from build123d import *

# Parameters (mm, degrees)
SKETCH1_R           = 44.45
BOSS_EXTRUDE1_DEPTH = 25.4
CHAMFER1_SIZE       = 10
SKETCH3_R           = 1.8161
CUT_EXTRUDE1_DEPTH  = 26.4
BOSS_EXTRUDE3_DEPTH = 50.8


with BuildPart() as part:
    # Sketch1 → Boss-Extrude1 (new body)
    with BuildSketch(Plane.XY):
        with BuildLine():
            ThreePointArc((67.188694676, -58.214167586), (88.9, 0), (67.188694676, 58.214167586))
            ThreePointArc((67.188694676, 58.214167586), (67.351920908, 67.351920908), (58.214167586, 67.188694676))
            ThreePointArc((58.214167586, 67.188694676), (0, 88.9), (-58.214167586, 67.188694676))
            ThreePointArc((-58.214167586, 67.188694676), (-67.351920908, 67.351920908), (-67.188694676, 58.214167586))
            ThreePointArc((-67.188694676, 58.214167586), (-88.9, 0), (-67.188694676, -58.214167586))
            ThreePointArc((-67.188694676, -58.214167586), (-67.351920908, -67.351920908), (-58.214167586, -67.188694676))
            ThreePointArc((-58.214167586, -67.188694676), (0, -88.9), (58.214167586, -67.188694676))
            ThreePointArc((58.214167586, -67.188694676), (67.351920908, -67.351920908), (67.188694676, -58.214167586))
        make_face()
        Circle(SKETCH1_R, mode=Mode.SUBTRACT)
    extrude(amount=BOSS_EXTRUDE1_DEPTH)

    # Chamfer1
    chamfer1_edges = [part.edges().sort_by_distance(p)[0] for p in [
        (-44.45, 0, 25.4),
    ]]
    chamfer(chamfer1_edges, length=CHAMFER1_SIZE)

    # Sketch3 → Cut-Extrude1 (cut, through all)
    with BuildSketch(Plane.XY.offset(25.4)):
        with Locations((61.065741623, 61.065741623)):
            Circle(SKETCH3_R)
        with Locations((61.065741623, -61.065741623)):
            Circle(SKETCH3_R)
        with Locations((-61.065741623, -61.065741623)):
            Circle(SKETCH3_R)
        with Locations((-61.065741623, 61.065741623)):
            Circle(SKETCH3_R)
    extrude(amount=-CUT_EXTRUDE1_DEPTH, mode=Mode.SUBTRACT)

    # Sketch5 → Boss-Extrude3 (add)
    with BuildSketch(Plane(origin=(0, 0, 0), x_dir=(-1, 0, 0), z_dir=(0, 0, -1))):
        with BuildLine():
            Line((-76.835, 12.7), (-56.515, 12.7))
            ThreePointArc((-56.515, 12.7), (-54.718948776, 11.956051224), (-53.975, 10.16))
            Line((-53.975, 10.16), (-53.975, -10.16))
            ThreePointArc((-53.975, -10.16), (-54.718948776, -11.956051224), (-56.515, -12.7))
            Line((-56.515, -12.7), (-76.835, -12.7))
            ThreePointArc((-76.835, -12.7), (-78.631051224, -11.956051224), (-79.375, -10.16))
            Line((-79.375, -10.16), (-79.375, 10.16))
            ThreePointArc((-79.375, 10.16), (-78.631051224, 11.956051224), (-76.835, 12.7))
        make_face()
        with BuildLine():
            Line((-10.16, -79.375), (10.16, -79.375))
            ThreePointArc((10.16, -79.375), (11.956051224, -78.631051224), (12.7, -76.835))
            Line((12.7, -76.835), (12.7, -56.515))
            ThreePointArc((12.7, -56.515), (11.956051224, -54.718948776), (10.16, -53.975))
            Line((10.16, -53.975), (-10.16, -53.975))
            ThreePointArc((-10.16, -53.975), (-11.956051224, -54.718948776), (-12.7, -56.515))
            Line((-12.7, -56.515), (-12.7, -76.835))
            ThreePointArc((-12.7, -76.835), (-11.956051224, -78.631051224), (-10.16, -79.375))
        make_face()
        with BuildLine():
            Line((12.7, 76.835), (12.7, 56.515))
            ThreePointArc((12.7, 56.515), (11.956051224, 54.718948776), (10.16, 53.975))
            Line((10.16, 53.975), (-10.16, 53.975))
            ThreePointArc((-10.16, 53.975), (-11.956051224, 54.718948776), (-12.7, 56.515))
            Line((-12.7, 56.515), (-12.7, 76.835))
            ThreePointArc((-12.7, 76.835), (-11.956051224, 78.631051224), (-10.16, 79.375))
            Line((-10.16, 79.375), (10.16, 79.375))
            ThreePointArc((10.16, 79.375), (11.956051224, 78.631051224), (12.7, 76.835))
        make_face()
        with BuildLine():
            Line((76.835, -12.7), (56.515, -12.7))
            ThreePointArc((56.515, -12.7), (54.718948776, -11.956051224), (53.975, -10.16))
            Line((53.975, -10.16), (53.975, 10.16))
            ThreePointArc((53.975, 10.16), (54.718948776, 11.956051224), (56.515, 12.7))
            Line((56.515, 12.7), (76.835, 12.7))
            ThreePointArc((76.835, 12.7), (78.631051224, 11.956051224), (79.375, 10.16))
            Line((79.375, 10.16), (79.375, -10.16))
            ThreePointArc((79.375, -10.16), (78.631051224, -11.956051224), (76.835, -12.7))
        make_face()
    extrude(amount=BOSS_EXTRUDE3_DEPTH)


solid = part.part
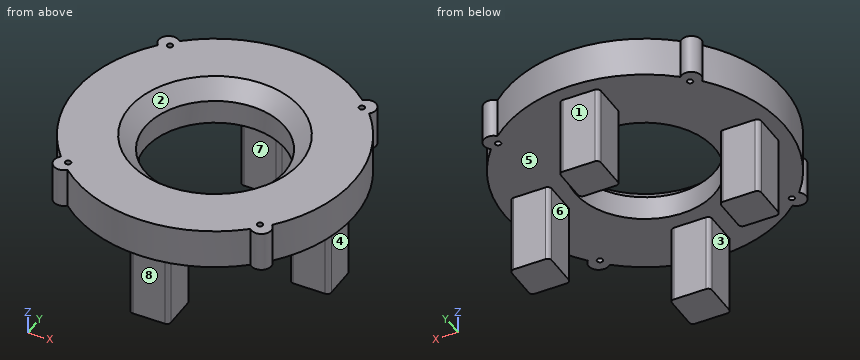
The model under review builds one solid part; all positions refer to its coordinate system, in mm. Face numbers are marked on the shaded views. A direction names the side the tool comes from. Give positions to 0.01 mm unless a question says otherwise; leave off trailing zeros. Loops run counter-clockwise (first coordinate to the right, second up) from the corner with the lowest first, then second, coordinate; pieces in that order, holes last. Notation, with made-up numbers: (-15, 37) -> (19, 37) arc R24 ccw to (19, 56) -> close; hole circle Ø9 at (-36, 37.25). An arc over 180 degrees is marked (long way). Put each result on its own line as item: value. Start each with the question number.
1. For the marked faces 1, 2, 3, 4 and 5, list the 3-axis set-ups (+Z, -Z, +X, -X, +Y, -Y) from which the entire face can be reached by the end or side of a thin tool; tool diameter is ignored.
2. Mouldability with a two-part tool opening along Y and no side actions: class the marked faces 6, 7 and 8 as released by +Y, released by -Y, zero draft, split by the parting line, or undercut.
3. Wall thickness on probe 1 along X at (y, z) = (4.5, -35) (3 decimals); probe 2 along X at (y, z) = (67, -21.5); probe 3 along Y at (x, z) = (-37, 1): over which ranges is each line inside the solid? List them lowest first.
4. We need section B-B on z = -13. State how many separate pieces and enclosed holes the cut face has, then the cut area to 3 significant figures.
5. We need section A-A on x = 0. State the section outline as (y, z) points (3 decimals), then the cut area to 3 significant figures.
6. Clearance check with flat-ended pins moving along their axes: P1, Ø6, axis at x = 3.5, z = -32, coming from the -Y side (3 decimals); P2, Ø4, axis at x = -61.07, y = -61.07, coming from the +Z side; P3, Ø6, axis at x = 70.5, z = -21.5, coming from the -Y side; P4, Ø6, axis at y = 2, z = -31.5, coming from the -X side (3 decimals). State where each tip first meets the part, or that it passes through.
Determined:
1. face 1: -Z, +X, -X, +Y
1. face 2: +Z
1. face 3: -Z, -X, +Y, -Y
1. face 4: -Z, +X, +Y, -Y
1. face 5: -Z
2. face 6: zero draft
2. face 7: undercut
2. face 8: released by -Y
3. probe 1: -79.375 to -53.975, 53.975 to 79.375
3. probe 2: -12.7 to 12.7
3. probe 3: -80.83 to -24.63, 24.63 to 80.83
4. separate pieces: 4
4. enclosed holes: 0
4. area: 2,560 mm^2
5. outline: (-88.9, 0) -> (-79.375, 0) -> (-79.375, -50.8) -> (-53.975, -50.8) -> (-53.975, 0) -> (-44.45, 0) -> (-44.45, 15.4) -> (-54.45, 25.4) -> (-88.9, 25.4) -> close; (44.45, 0) -> (53.975, 0) -> (53.975, -50.8) -> (79.375, -50.8) -> (79.375, 0) -> (88.9, 0) -> (88.9, 25.4) -> (54.45, 25.4) -> (44.45, 15.4) -> close
5. area: 4,740 mm^2
6. P1: y = -79.375
6. P2: z = 25.4
6. P3: y = -12.7
6. P4: x = -79.375
